Could you check a few things on this model? Use its own coordinates, in mm. A direction names the side the tool comes from. Round coordinates to 2 decimals unless told otherwise and drop trailing zeros. Order: outer loops, then holes, each group sorted by start corner. A loop starts at its lowest first (then second) coordinate and runs counter-clockwise, first axis right, second up. Notation, with made-up numbers: (22, 15.25) - (33, 15.25) arc R20 ccw to (33, 50.25) - close; hole circle Ø7 at (29, -25). An arc over 180 degrees is marked (long way). Return JSON: item names as keys, results as strings. Group by question number.
from build123d import *

# Parameters (mm, degrees)
SKETCH1_W           = 12.5
SKETCH1_H           = 2.5
SKETCH1_W_2         = 2.5
SKETCH1_H_2         = 12.5
SKETCH1_W_3         = 9
SKETCH1_H_3         = 6
BOSS_EXTRUDE1_DEPTH = 3
FILLET1_R           = 2
SKETCH1_6_R         = 2.5
SKETCH1_6_R_2       = 1.25
BOSS_EXTRUDE4_DEPTH = 23
SKETCH3_R           = 1
CUT_EXTRUDE1_DEPTH  = 10


with BuildPart() as part:
    # Sketch1 → Boss-Extrude1 (new body)
    with BuildSketch(Plane(origin=(0, 0, 0), x_dir=(1, 0, 0), z_dir=(0, 1, 0))):
        Polygon((-14.041444449, -20.13144272), (-14.041444449, -12.640037485), (-38.561763486, -12.640037485), (-38.561763486, -34.640037485), (-1.270220731, -34.640037485), (-1.270220731, -12.640037485), (-4.270220731, -12.640037485), (-4.270220731, -20.13144272), align=None)
        with Locations((-10.520220731, -30.890037485)):
            Rectangle(SKETCH1_W, SKETCH1_H, mode=Mode.SUBTRACT)
        with Locations((-34.020220731, -25.190037485)):
            Rectangle(SKETCH1_W_2, SKETCH1_H_2, mode=Mode.SUBTRACT)
        with Locations((-24.475907507, -25.190037485)):
            Rectangle(SKETCH1_W_3, SKETCH1_H_3, mode=Mode.SUBTRACT)
    extrude(amount=BOSS_EXTRUDE1_DEPTH)

    # Fillet1
    fillet1_edges = [part.edges().sort_by_distance(p)[0] for p in [
        (-14.041444449, 1.5, 20.13144272),
        (-4.270220731, 1.5, 20.13144272),
        (-1.270220731, 1.5, 34.640037485),
        (-38.561763486, 1.5, 34.640037485),
        (-38.561763486, 1.5, 12.640037485),
    ]]
    fillet(fillet1_edges, radius=FILLET1_R)

    # Sketch1_6 → Boss-Extrude4 (add)
    # profile 1 of 4: a face of its own
    with BuildSketch(Plane(origin=(0, 0, 0), x_dir=(1, 0, 0), z_dir=(0, 1, 0))):
        with Locations(Location((-19.270220731, -32.140037485, 0), (0, 0, 270))):
            Circle(SKETCH1_6_R)
        with Locations((-19.270220731, -32.140037485)):
            Circle(SKETCH1_6_R_2, mode=Mode.SUBTRACT)
    # profile 2 of 4: a face of its own
    with BuildSketch(Plane(origin=(0, 0, 0), x_dir=(1, 0, 0), z_dir=(0, 1, 0))):
        with Locations(Location((-19.270220731, -15.140037485, 0), (0, 0, 270))):
            Circle(SKETCH1_6_R)
        with Locations((-19.270220731, -15.140037485)):
            Circle(SKETCH1_6_R_2, mode=Mode.SUBTRACT)
    # profile 3 of 4: a face of its own
    with BuildSketch(Plane(origin=(0, 0, 0), x_dir=(1, 0, 0), z_dir=(0, 1, 0))):
        with Locations((-19.270220731, -15.140037485)):
            Circle(SKETCH1_6_R_2)
    # profile 4 of 4: a face of its own
    with BuildSketch(Plane(origin=(0, 0, 0), x_dir=(1, 0, 0), z_dir=(0, 1, 0))):
        with Locations((-19.270220731, -32.140037485)):
            Circle(SKETCH1_6_R_2)
    extrude(amount=-BOSS_EXTRUDE4_DEPTH)

    # Sketch3 → Cut-Extrude1 (cut)
    with BuildSketch(Plane(origin=(0, -23, 0), x_dir=(-1, 0, 0), z_dir=(0, -1, 0))):
        with Locations(Location((19.270220731, -32.140037485, 0), (0, 0, 90))):
            Circle(SKETCH3_R)
        with Locations(Location((19.270220731, -15.140037485, 0), (0, 0, 90))):
            Circle(SKETCH3_R)
    extrude(amount=-CUT_EXTRUDE1_DEPTH, mode=Mode.SUBTRACT)


solid = part.part
1) If I drill on line 1 along X through (y, z) = (1, 27.5); line 2 along Y through (x, z) = (-32, 33.5); line 3 along Y through (x, z) = (-20, 31.5), over which ranges is the centre line in solid material (lowest first)? Write a range as from..to.
2) For faces 4 (the flat face through (-3, 1, 12.64)), 5 (the flat face through (-4.27, 1, 31)), 6 (the flat face through (-20.3, -23, 15.7)), 7 (the flat face through (-4.27, 1, 15)), 8 (the cylindrical face through (-20.16, -18.07, 31.68)), which set-ups out of +Z, -Z, +X, -X, +Y, -Y let a thin tool reach every point of the face, with its end or its side?
3) We'd pull the mould along X, two halves only. Please class faces 1 (the flat face through (-20.3, -23, 32.7)), 2 (the cylindrical face through (-13.5, 1.5, 19.5)), 3 (the cylindrical face through (-1.87, 1.52, 34.07)): +X half, -X half, draft (parallel to the pull), parting line (faces both ways), or undercut.
4) I want a section at D-D, the plane x = -16. List the corners of the cut face in (y, z) for me, plus the area to 3 significant figures.
5) I want a section at A-A, the plane x = -28. List the corners of the cut face in (y, z) for me, plus the area to 3 significant figures.
6) I want a section at B-B, the plane z = 22.75. List the corners of the cut face in (x, y) for me, plus the area to 3 significant figures.
7) Will these pins go through, and if not, where does the flat tip stop? pin 1 (6 mm diameter, centred on y = -14.5, z = 28, fed in from +X); pin 2 (3 mm diameter, centred on x = -14.5, z = 17.5, fed in from -Y); pin 3 (0.6 mm diameter, centred on x = -19.5, z = 32.5, fed in from -Y).
8) I want a section at C-C, the plane y = 1.25. List the corners of the cut face in (x, z) for me.
Outcome:
{
 "1": {"line 1": "-38.56..-35.27, -32.77..-28.98, -19.98..-1.27", "line 2": "0..3", "line 3": "-13..3"},
 "2": {"face 4": "-Z, +X, -X, +Y, -Y", "face 5": "+Y, -Y", "face 6": "+Z, -Z, +X, -X, -Y", "face 7": "-Z, +Y, -Y", "face 8": "-Y"},
 "3": {"face 1": "draft", "face 2": "undercut", "face 3": "+X half"},
 "4": {"outline": "(0, 12.64) - (3, 12.64) - (3, 29.64) - (0, 29.64) - close; (0, 32.14) - (3, 32.14) - (3, 34.64) - (0, 34.64) - close", "area": "58.5 mm^2"},
 "5": {"outline": "(0, 12.64) - (3, 12.64) - (3, 22.19) - (0, 22.19) - close; (0, 28.19) - (3, 28.19) - (3, 34.64) - (0, 34.64) - close", "area": "48.0 mm^2"},
 "6": {"outline": "(-38.56, 0) - (-35.27, 0) - (-35.27, 3) - (-38.56, 3) - close; (-32.77, 0) - (-28.98, 0) - (-28.98, 3) - (-32.77, 3) - close; (-19.98, 0) - (-1.27, 0) - (-1.27, 3) - (-19.98, 3) - close", "area": "77.4 mm^2"},
 "7": {"pin 1": "x = -17.05", "pin 2": "y = 0", "pin 3": "y = -13"},
 "8": {"outline": "(-38.56, 14.64) arc R2 ccw to (-36.56, 12.64) - (-14.04, 12.64) - (-14.04, 18.13) arc R2 cw to (-12.04, 20.13) - (-6.27, 20.13) arc R2 cw to (-4.27, 18.13) - (-4.27, 12.64) - (-1.27, 12.64) - (-1.27, 32.64) arc R2 ccw to (-3.27, 34.64) - (-36.56, 34.64) arc R2 ccw to (-38.56, 32.64) - close; hole (-35.27, 18.94) - (-32.77, 18.94) - (-32.77, 31.44) - (-35.27, 31.44) - close; hole (-28.98, 22.19) - (-19.98, 22.19) - (-19.98, 28.19) - (-28.98, 28.19) - close; hole (-16.77, 29.64) - (-4.27, 29.64) - (-4.27, 32.14) - (-16.77, 32.14) - close"}
}
